Could you check a few things on this model? Use its own coordinates, in mm. Coordinates: 2 decimals unless noted, no trailing zeros. Order: outer loops, then holes, each group sorted by start corner. A loop starts at its lowest first (then second) coordinate and runs counter-clockwise, first axis right, second up. Notation, with made-up numbers: (-23, 33.25) -> (7, 33.25) arc R30 cw to (7, 72.25) -> close; hole circle Ø7 at (60, 46.25). An arc over 180 degrees is marked (long way). Put each result on its own line as item: value. Start each with the question number.
Q1. Will these pins go through, and if not, where does the flat tip stop? pin 1 (2 mm diameter, centred on x = -20.5, y = 23, fed in from -Z); pin 2 (3 mm diameter, centred on x = 20.5, z = -7.5, fed in from -Y); pin 3 (2 mm diameter, centred on y = -20, z = 3.5, fed in from +X); pin 4 (16 mm diameter, centred on x = 0, y = 0, fed in from +Z).
Q2. Please list where these lines run through material, in increasing order: line 1 along X through (y, z) = (-0.5, 4); line 2 along Y through (x, z) = (0, -6); line 3 along Y through (x, z) = (-7.5, -3.75).
Q3. If we section it at A-A (y = 0): Please give me the cut outline in (x, z).
Q4. If we section it at D-D (z = -4.5): Please give me the cut outline in (x, y).
Q5. If we section it at C-C (z = 14.75): Please give me the cut outline in (x, y).
Q6. We'd pull the mould along X, two halves only. Please class faces 1 (the face through (-2.202, -9.915, 14.156)), 2 (the face through (-21.919, -16.807, 16.379)), 3 (the face through (6, -12, 16.5)): +X half, -X half, draft (parallel to the pull), parting line (faces both ways), or undercut.
from build123d import *

# Parameters (mm, degrees)
SKETCH1_R           = 3
SKETCH1_R_2         = 1
EXTRUDE_THIN1_DEPTH = 3
CHAMFER1_SIZE       = 0.25
SCALE1_SCALE        = 10


with BuildPart() as part:
    # Sketch1 → Extrude-Thin1 (new body)
    with BuildSketch(Plane.XY):
        Circle(SKETCH1_R)
        Circle(SKETCH1_R_2, mode=Mode.SUBTRACT)
    extrude(amount=EXTRUDE_THIN1_DEPTH)

    # Chamfer1
    chamfer1_edges = [part.edges().sort_by_distance(p)[0] for p in [
        (-3, 0, 0),
        (-1, 0, 0),
        (-3, 0, 3),
        (-1, 0, 3),
    ]]
    chamfer(chamfer1_edges, length=CHAMFER1_SIZE)


with BuildPart() as part_1:
    # Scale1: scaled about (0, 0, 1.5)
    add(part.part.scale(SCALE1_SCALE).moved(Location((0, 0, -13.5))))


solid = part_1.part
The answers:
1. pin 1: z = -11.19
1. pin 2: y = -23.22
1. pin 3: x = 23.22
1. pin 4: through
2. line 1: -30 to -9.99, 9.99 to 30
2. line 2: -30 to -10, 10 to 30
2. line 3: -29.05 to -6.61, 6.61 to 29.05
3. outline: (-30, -11) -> (-27.5, -13.5) -> (-12.5, -13.5) -> (-10, -11) -> (-10, 14) -> (-12.5, 16.5) -> (-27.5, 16.5) -> (-30, 14) -> close; (10, -11) -> (12.5, -13.5) -> (27.5, -13.5) -> (30, -11) -> (30, 14) -> (27.5, 16.5) -> (12.5, 16.5) -> (10, 14) -> close
4. outline: circle Ø60 at (0, 0); hole circle Ø20 at (0, 0)
5. outline: circle Ø58.5 at (0, 0); hole circle Ø21.5 at (0, 0)
6. face 1: undercut
6. face 2: parting line
6. face 3: draft
